Autodesk Inventor part; units mm, degrees
ref_plane "YZ Plane" through (0, 0, 0) normal (1, 0, 0) x (0, 1, 0)
ref_plane "XZ Plane" through (0, 0, 0) normal (0, 1, 0) x (-1, 0, 0)
ref_plane "XY Plane" through (0, 0, 0) normal (0, 0, 1) x (1, 0, 0)
sketch "Szkic1" plane through (0, 0, 0) normal (0, 0, 1) x (1, 0, 0)
  line L0 (2.6774, 0.115) -> (-0.6, 0.115)
  spline S0 degree 3 poles (3.0833, -0.1968) (3.1541, -0.2257) (3.223, -0.256) (3.5835, -0.4251) (3.888, -0.6087) (4.4504, -1.0382) (4.7087, -1.2836) (5.1613, -1.7912) (5.3932, -2.1042) (5.7913, -2.77) (5.9577, -3.1227) (6.2121, -3.7972) (6.3223, -4.1828) (6.4663, -4.968) (6.5, -5.3675) (6.5, -5.7331) knots -1.428143 -1.428143 -1.428143 -1.428143 -1.406087 -1.406087 -1.308684 -1.308684 -1.211282 -1.211282 -1.104676 -1.104676 -0.99807 -0.99807 -0.888411 -0.888411 -0.778752 -0.778752 -0.778752 -0.778752
  line L1 (6.5, -5.7331) -> (6.5, -13.1255)
  circle A0 centre (3.25, -5.9055) radius 1.5
  line L2 (-0.6, 0) -> (-0.6, -13.1255)
  line L3 (-0.6, -13.4271) -> (99.4, -13.4271)
  line L4 (-0.6, -14.1019) -> (-0.6, -13.1255)
  line L5 (6.5, -14.1019) -> (6.5, -13.1255)
  line L6 (-0.6, -13.4271) -> (-0.6, -28.9827)
  line L7 (-0.6, -13.4271) -> (-0.6, -28.9827)
  line L8 (-0.6, -13.4271) -> (99.4, -13.4271)
  line L9 (99.4, -13.4271) -> (99.4, 3.0729)
  line L10 (99.4, 3.0729) -> (-0.6, 3.0729)
  line L11 (-0.6, 3.0729) -> (-0.6, -13.4271)
  point P0 (0, 0)
  dimension "d0" = 16.5
extrude "Wyciągnięcie proste1" add sketch "Szkic1" along normal blind 2 contours A0 | L11 L10 L9 L3 L4 L2
sketch "Szkic2" plane through (0, 0, 2) normal (0, 0, 1) x (1, 0, 0)
  line L0 (79.4, 9.1073) -> (19.4, 9.1073)
  line L1 (99.4, 3.0729) -> (-0.6, 3.0729)
  line L2 (79.4, 9.1073) -> (19.4, 9.1073)
  line L3 (19.4, 9.1073) -> (19.4, 3.0729)
  line L4 (19.4, 3.0729) -> (79.4, 3.0729)
  line L5 (79.4, 3.0729) -> (79.4, 9.1073)
  point P0 (0, 0)
extrude "Wyciągnięcie proste2" add sketch "Szkic2" against normal up to surface (2 mm away)
sketch "Szkic3" plane through (0, 0, 2) normal (0, 0, 1) x (1, 0, 0)
  line L0 (99.4, -13.4271) -> (99.4, 3.0729)
  line L1 (99.4, 3.0729) -> (79.4, 3.0729)
  line L2 (79.4, 3.0729) -> (79.4, 9.1073)
  line L3 (79.4, 9.1073) -> (19.4, 9.1073)
  line L4 (19.4, 9.1073) -> (19.4, 3.0729)
  line L5 (19.4, 3.0729) -> (-0.6, 3.0729)
  line L6 (-0.6, 3.0729) -> (-0.6, -13.4271)
  line L7 (-0.6, -13.4271) -> (99.4, -13.4271)
  line L8 (79.4, 9.1073) -> (19.4, 9.1073)
  line L9 (19.4, 9.1073) -> (19.4, 26.1073)
  line L10 (19.4, 26.1073) -> (79.4, 26.1073)
  line L11 (79.4, 26.1073) -> (79.4, 9.1073)
  point P0 (0, 0)
  dimension "d5" = 17
extrude "Wyciągnięcie proste3" add sketch "Szkic3" against normal blind 2 contours L3 L9 L10 L11
sketch "Szkic4" plane through (0, 0, 2) normal (0, 0, 1) x (1, 0, 0)
  circle A0 centre (3.25, -5.9055) radius 1.5
  line L0 (79.4, 26.1073) -> (19.4, 26.1073)
  line L1 (19.4, 26.1073) -> (79.4, 26.1073)
  line L2 (49.4, 26.1073) -> (49.4, -13.4271)
  line L3 (-0.6, -13.4271) -> (99.4, -13.4271)
  circle A1 centre (95.55, -5.9055) radius 1.5
  point P0 (0, 0)
extrude "Wyciągnięcie proste4" cut sketch "Szkic4" against normal through all
sketch "Szkic5" plane through (0, 0, 2) normal (0, 0, 1) x (1, 0, 0)
  line L0 (-0.6, -13.4271) -> (99.4, -13.4271)
  line L1 (-0.6, 3.0729) -> (-0.6, -13.4271)
  line L2 (-0.6, -13.4271) -> (99.4, -13.4271)
  line L3 (99.4, -13.4271) -> (99.4, -14.4271)
  line L4 (99.4, -14.4271) -> (-0.6, -14.4271)
  line L5 (-0.6, -14.4271) -> (-0.6, -13.4271)
  point P0 (0, 0)
  dimension "d10" = 1
extrude "Wyciągnięcie proste5" add sketch "Szkic5" against normal up to surface (2 mm away)
properties part number "tylna"
Here's how the part is built. I have some questions about the finished solid (model axes, mm). A direction names the side the tool comes from. Coordinates: 2 decimals unless noted, no trailing zeros. Write each loop counter-clockwise with the first axis right and the second up, starting at its lowest first coordinate (ties: lowest second). Pieces come first, ordered by that corner, then holes. Notation, with made-up numbers: (5.5, 13) -> (56.5, 13) arc R26 cw to (56.5, 44) -> close; hole circle Ø1 at (5, 41). An arc over 180 degrees is marked (long way). Use a Markdown table: item, result. Add a question column.
(1) For faces 5 (the flat face through (19.4, 14, 1)), 6 (the flat face through (79.4, 15, 1)), 7 (the flat face through (-0.6, -6, 1)), which set-ups out of +Z, -Z, +X, -X, +Y, -Y let a thin tool reach every point of the face, with its end or its side?
(2) Please list where these lines run through material, in increasing order: line 1 (X direction, y = -6, z = 1.85); line 2 (Y direction, x = 95.55, z = 1.6); line 3 (X direction, y = 18, z = 1.85).
(3) If we section it at A-A, the plane x = 3.25: Write out the boundary of the cut face in (y, z), and give its area (3 significant figures).
(4) If we section it at B-B, the plane z = 1.25: Write out the boundary of the cut face in (x, y), and give its area (3 significant figures).
(5) If we section it at C-C, the plane y = 20: Write out the boundary of the cut face in (x, z), and give its area (3 significant figures).
(6) We'd pull the mould along Y, two halves only. Please class faces 1 (the cylindrical face through (96.242, -7.236, 1.014)), 2 (the flat face through (50, -14.427, 1)), 3 (the cylindrical face through (3.942, -7.236, 1.014)), 4 (the flat face through (49, 26.107, 1)): +Y half, -Y half, draft (parallel to the pull), parting line (faces both ways), or undercut.
(7) I'm going to push flat-ended pins straight in: P1, Ø6, axis at x = 27.5, y = -4, coming from the -Z side; P2, Ø0.6, axis at x = 4.5, z = 0.5, coming from the +Y side; P3, Ø0.6, axis at y = 12.5, z = 0.5, coming from the +X side; P4, Ø2.5, axis at x = 95.55, y = -5.91, coming from the -Z side. Where does each tip first touch, or does it pass through?
Outcome:
| question | item | result |
|---|---|---|
| 1 | face 5 | +Z, -Z, -X, +Y |
| 1 | face 6 | +Z, -Z, +X, +Y |
| 1 | face 7 | +Z, -Z, -X, +Y, -Y |
| 2 | line 1 | x = -0.6 to 1.75, 4.75 to 94.05, 97.05 to 99.4 |
| 2 | line 2 | y = -14.43 to -7.41, -4.41 to 3.07 |
| 2 | line 3 | x = 19.4 to 79.4 |
| 3 | outline | (-14.43, 0) -> (-7.41, 0) -> (-7.41, 2) -> (-14.43, 2) -> close; (-4.41, 0) -> (3.07, 0) -> (3.07, 2) -> (-4.41, 2) -> close |
| 3 | area | 29.0 mm^2 |
| 4 | outline | (-0.6, -14.43) -> (99.4, -14.43) -> (99.4, 3.07) -> (79.4, 3.07) -> (79.4, 26.11) -> (19.4, 26.11) -> (19.4, 3.07) -> (-0.6, 3.07) -> close; hole circle Ø3 at (3.25, -5.91); hole circle Ø3 at (95.55, -5.91) |
| 4 | area | 3,120 mm^2 |
| 5 | outline | (19.4, 0) -> (79.4, 0) -> (79.4, 2) -> (19.4, 2) -> close |
| 5 | area | 120 mm^2 |
| 6 | face 1 | undercut |
| 6 | face 2 | -Y half |
| 6 | face 3 | undercut |
| 6 | face 4 | +Y half |
| 7 | P1 | stops at z = 0 |
| 7 | P2 | stops at y = 3.07 |
| 7 | P3 | stops at x = 79.4 |
| 7 | P4 | passes through |
